```python
from build123d import *

# Parameters (mm, degrees)
SKETCH_2_W      = 25.0000008
SKETCH_2_H      = 15.04999784
EXTRUDE_2_DEPTH = 24
SKETCH_3_R      = 0.75
SKETCH_3_R_2    = 0.5
EXTRUDE_3_DEPTH = 5


with BuildPart() as part:
    # Эскиз2 → Бобышка-Вытянуть2 (new body)
    with BuildSketch(Plane.XY):
        with Locations((-17.07912528, 17.543231945)):
            Rectangle(SKETCH_2_W, SKETCH_2_H)
    extrude(amount=EXTRUDE_2_DEPTH)

    # Эскиз3 → Бобышка-Вытянуть3 (add)
    with BuildSketch(Plane(origin=(0, 0, 0), x_dir=(-1, 0, 0), z_dir=(0, 0, -1))):
        with Locations(Location((6.77912488, 12.218233025, 0), (0, 0, 180))):
            Circle(SKETCH_3_R)
        with Locations(Location((11.07912488, 14.568230865, 0), (0, 0, 180))):
            Circle(SKETCH_3_R_2)
        with Locations(Location((17.07912558, 14.568230865, 0), (0, 0, 180))):
            Circle(SKETCH_3_R_2)
        with Locations(Location((11.07912488, 20.568230865, 0), (0, 0, 180))):
            Circle(SKETCH_3_R_2)
        with Locations(Location((17.07912558, 20.568230865, 0), (0, 0, 180))):
            Circle(SKETCH_3_R_2)
        with Locations(Location((23.07912628, 20.568230865, 0), (0, 0, 180))):
            Circle(SKETCH_3_R_2)
        with Locations(Location((23.07912628, 14.568230865, 0), (0, 0, 180))):
            Circle(SKETCH_3_R_2)
        with Locations(Location((27.37912568, 12.218233025, 0), (0, 0, 180))):
            Circle(SKETCH_3_R)
    extrude(amount=EXTRUDE_3_DEPTH)


solid = part.part
```
Could you check a few things on this model? Use its own coordinates, in mm. A direction names the side the tool comes from. Round coordinates to 2 decimals unless told otherwise and drop trailing zeros. Loops run counter-clockwise (first coordinate to the right, second up) from the corner with the lowest first, then second, coordinate; pieces in that order, holes last. Notation, with made-up numbers: (64.5, 86.25) - (122.5, 86.25) arc R11 ccw to (122.5, 105.25) - close; hole circle Ø9 at (-32, 2). An arc over 180 degrees is marked (long way). Answer in a Markdown table with one row per item. Add a question column.
(1) If we section it at A-A (y = 17.5): Please give me the cut outline in (x, z), plus the area to 3 significant figures.
(2) If we section it at C-C (x = -18.75): Please give me the cut outline in (y, z), plus the area to 3 significant figures.
(3) I need wall thicknesses on line 1 along Z through (x, y) = (-23.5, 17.75). Which ranges of the line are inside material? Lowest first, please.
(4) For faces 5 (the face through (-16.617, 14.76, -2.465)), 6 (the face through (-11.1, 14.6, -5)), which set-ups out of +Z, -Z, +X, -X, +Y, -Y let a thin tool reach every point of the face, with its end or its side?
(5) If we mould it in two halves opening along Y, with no side actions, what happens to faces 1 (the face through (-4.579, 17, 12)), 2 (the face through (-17, 25.068, 12)), 3 (the face through (-6.43, 12.88, -2.46)), 4 (the face through (-23.48, 14.87, -2.46))? For each: pulls with the +Y half, pulls with the -Y half, needs draft (parallel to the pull), parting line crosses it, or undercut.
(6) If we section it at B-B (x = -7): Please give me the cut outline in (y, z), plus the area to 3 significant figures.
Model answer:
| question | item | result |
|---|---|---|
| 1 | outline | (-29.58, 0) - (-4.58, 0) - (-4.58, 24) - (-29.58, 24) - close |
| 1 | area | 600 mm² |
| 2 | outline | (10.02, 0) - (25.07, 0) - (25.07, 24) - (10.02, 24) - close |
| 2 | area | 361 mm² |
| 3 | line 1 | z = 0 to 24 |
| 4 | face 5 | -Z |
| 4 | face 6 | -Z, +X, -X, +Y, -Y |
| 5 | face 1 | needs draft |
| 5 | face 2 | pulls with the +Y half |
| 5 | face 3 | parting line crosses it |
| 5 | face 4 | undercut |
| 6 | outline | (10.02, 0) - (11.5, 0) - (11.5, -5) - (12.93, -5) - (12.93, 0) - (25.07, 0) - (25.07, 24) - (10.02, 24) - close |
| 6 | area | 368 mm² |
